For this review, take the finished solid that the model builds, in its own axes (mm). A direction names the side the tool comes from. Give positions to 0.01 mm unless a question says otherwise; leave off trailing zeros. Order: outer loops, then holes, each group sorted by start corner. A loop starts at its lowest first (then second) coordinate and runs counter-clockwise, first axis right, second up. Notation, with made-up numbers: (4, 52) - (28, 52) arc R31 ccw to (28, 80) - close; hole circle Ø2 at (63, 59.5). An arc over 180 degrees is marked (long way). Answer as a JSON object with one key per item and string values. Group by question number.
from build123d import *

# Parameters (mm, degrees)
SKETCH1_W           = 25
SKETCH1_H           = 84
SKETCH1_R           = 1.75
SKETCH1_W_2         = 4.7625
SKETCH1_H_2         = 5.6
BOSS_EXTRUDE1_DEPTH = 4.7625


with BuildPart() as part:
    # Sketch1 → Boss-Extrude1 (new body)
    with BuildSketch(Plane(origin=(0, 0, 0), x_dir=(1, 0, 0), z_dir=(0, 1, 0))):
        with Locations((12.5, 42)):
            Rectangle(SKETCH1_W, SKETCH1_H)
        with Locations((12.5, 10)):
            Circle(SKETCH1_R, mode=Mode.SUBTRACT)
        with Locations((12.5, 42)):
            Circle(SKETCH1_R, mode=Mode.SUBTRACT)
        with Locations((12.5, 74)):
            Circle(SKETCH1_R, mode=Mode.SUBTRACT)
        with Locations((27.38125, 30.8)):
            Rectangle(SKETCH1_W_2, SKETCH1_H_2)
        with Locations((27.38125, 19.6)):
            Rectangle(SKETCH1_W_2, SKETCH1_H_2)
        with Locations((27.38125, 42)):
            Rectangle(SKETCH1_W_2, SKETCH1_H_2)
        with Locations((27.38125, 53.2)):
            Rectangle(SKETCH1_W_2, SKETCH1_H_2)
        with Locations((27.38125, 64.4)):
            Rectangle(SKETCH1_W_2, SKETCH1_H_2)
        with Locations((27.38125, 75.6)):
            Rectangle(SKETCH1_W_2, SKETCH1_H_2)
        with Locations((27.38125, 8.4)):
            Rectangle(SKETCH1_W_2, SKETCH1_H_2)
    extrude(amount=BOSS_EXTRUDE1_DEPTH)


solid = part.part
1) For line 1 (Z direction, x = 12.5, y = 3.6); line 2 (Z direction, x = 11.5, y = 2.9); line 3 (X direction, y = 2.2, z = -74), list the stretches that pass through material, from the lowest coordinate up.
2) For pin 1 (3 mm diameter, centred on x = 12.5, z = -42, fed in from +Y); pin 2 (1.4 mm diameter, centred on y = 2.5, z = -82.5, fed in from +X); pin 3 (2.5 mm diameter, centred on x = 27.5, y = 3, fed in from +Z); pin 4 (1.4 mm diameter, centred on x = 27, y = 3.5, fed in from -Z), all flat-tipped, find the tip position at first contact; note any pin that passes through.
3) Consider section D-D (z = -14). Give the boundary of the cut face in (x, y).
4) Mouldability with a two-part tool opening along X and no side actions: class faces 4 (the face through (12.12, 2.35, -72.29)), 5 (the face through (25, 2, -36)), 6 (the face through (13.4, 2.3, -11.5)), 7 (the face through (12, 2, -84)) as released by +X, released by -X, zero draft, split by the parting line, or undercut.
5) Consider section C-C (y = 0.95). Give the number of separate pieces and of enclosed holes in the cut face, plus the area to 3 significant figures.
6) Consider section A-A (z = -42). Give the boundary of the cut face in (x, y), plus the area to 3 significant figures.
7) For faces 1 (the face through (25, 2, -3)), 2 (the face through (27, 2, -28)), 3 (the face through (27, 2, -78.4)), list the 3-axis set-ups (+Z, -Z, +X, -X, +Y, -Y) from which the entire face can be reached by the end or side of a thin tool; tool diameter is ignored.
8) Consider section B-B (x = 12.75). Give the boundary of the cut face in (y, z), plus the area to 3 significant figures.
Result set:
{
 "1": {"line 1": "z = -84 to -75.75, -72.25 to -43.75, -40.25 to -11.75, -8.25 to 0", "line 2": "z = -84 to -75.44, -72.56 to -43.44, -40.56 to -11.44, -8.56 to 0", "line 3": "x = 0 to 10.75, 14.25 to 29.76"},
 "2": {"pin 1": "passes through", "pin 2": "stops at x = 25", "pin 3": "stops at z = -5.6", "pin 4": "stops at z = -78.4"},
 "3": {"outline": "(0, 0) - (25, 0) - (25, 4.76) - (0, 4.76) - close"},
 "4": {"face 4": "undercut", "face 5": "released by +X", "face 6": "undercut", "face 7": "zero draft"},
 "5": {"separate pieces": "1", "enclosed holes": "3", "area": "2,260 mm2"},
 "6": {"outline": "(0, 0) - (10.75, 0) - (10.75, 4.76) - (0, 4.76) - close; (14.25, 0) - (29.76, 0) - (29.76, 4.76) - (14.25, 4.76) - close", "area": "125 mm2"},
 "7": {"face 1": "+Z, +X, +Y, -Y", "face 2": "+X, +Y, -Y", "face 3": "-Z, +X, +Y, -Y"},
 "8": {"outline": "(0, -84) - (4.76, -84) - (4.76, -75.73) - (0, -75.73) - close; (0, -72.27) - (4.76, -72.27) - (4.76, -43.73) - (0, -43.73) - close; (0, -40.27) - (4.76, -40.27) - (4.76, -11.73) - (0, -11.73) - close; (0, -8.27) - (4.76, -8.27) - (4.76, 0) - (0, 0) - close", "area": "351 mm2"}
}
